```python
from build123d import *

# Parameters (mm, degrees)
SKETCH_W        = 65
SKETCH_H        = 32
SKETCH_R        = 1.75
SKETCH_W_2      = 28
SKETCH_H_2      = 20
SKETCH_W_3      = 15.3
SKETCH_H_3      = 21
PAD_DEPTH       = 14
SKETCH001_W     = 63
SKETCH001_H     = 30
POCKET_DEPTH    = 11
SKETCH002_W     = 6.174751
SKETCH002_H     = 9.5
POCKET001_DEPTH = 7
SKETCH004_W     = 2
SKETCH004_H     = 20
PAD001_DEPTH    = 2
SKETCH005_W     = 15
SKETCH005_H     = 4
POCKET002_DEPTH = 5
SKETCH003_W     = 53
SKETCH003_H     = 5.2
POCKET003_DEPTH = 32.0010000001


with BuildPart() as part:
    # Sketch → Pad (new body)
    with BuildSketch(Plane.XY):
        with Locations((32.5, 16)):
            Rectangle(SKETCH_W, SKETCH_H)
        with Locations((3.5, 28.5)):
            Circle(SKETCH_R, mode=Mode.SUBTRACT)
        with Locations((61.4999634499, 28.5)):
            Circle(SKETCH_R, mode=Mode.SUBTRACT)
        with Locations((3.5, 3.5)):
            Circle(SKETCH_R, mode=Mode.SUBTRACT)
        with Locations((61.4999634499, 3.5)):
            Circle(SKETCH_R, mode=Mode.SUBTRACT)
        with Locations((41.4999634499, 16.7655958753)):
            Rectangle(SKETCH_W_2, SKETCH_H_2, mode=Mode.SUBTRACT)
        with Locations((14.8499634499, 17.4539391628)):
            Rectangle(SKETCH_W_3, SKETCH_H_3, mode=Mode.SUBTRACT)
    extrude(amount=PAD_DEPTH)

    # Sketch001 → Pocket (cut)
    with BuildSketch(Plane(origin=(0, 0, 0), x_dir=(1, 0, 0), z_dir=(0, 0, -1))):
        with Locations((32.5, -16)):
            Rectangle(SKETCH001_W, SKETCH001_H)
    extrude(amount=-POCKET_DEPTH, mode=Mode.SUBTRACT)

    # Sketch002 → Pocket001 (cut)
    with BuildSketch(Plane.XY.offset(14)):
        with Locations((61.9126245, 16)):
            Rectangle(SKETCH002_W, SKETCH002_H)
    extrude(amount=-POCKET001_DEPTH, mode=Mode.SUBTRACT)

    # Sketch004 → Pad001 (new body)
    with BuildSketch(Plane(origin=(0, 0, 11), x_dir=(1, 0, 0), z_dir=(0, 0, -1))):
        with Locations((26.4999634499, -16.7655958753)):
            Rectangle(SKETCH004_W, SKETCH004_H)
        with Locations((56.4999634499, -16.7655958753)):
            Rectangle(SKETCH004_W, SKETCH004_H)
    extrude(amount=PAD001_DEPTH)

    # Sketch005 → Pocket002 (cut)
    with BuildSketch(Plane(origin=(0, 0, 0), x_dir=(0, -1, 0), z_dir=(-1, 0, 0))):
        with Locations((-15.5, 5)):
            Rectangle(SKETCH005_W, SKETCH005_H)
    extrude(amount=-POCKET002_DEPTH, mode=Mode.SUBTRACT)

    # Sketch003 → Pocket003 (cut, through all)
    with BuildSketch(Plane(origin=(0, 32, 0), x_dir=(-1, 0, 0), z_dir=(0, 1, 0))):
        with Locations((-32.5, 6.4)):
            Rectangle(SKETCH003_W, SKETCH003_H)
    extrude(amount=-POCKET003_DEPTH, mode=Mode.SUBTRACT)


solid = part.part
```
Read the model definition and answer for the solid it produces. Units are mm, in the model's axes. A direction names the side the tool comes from. Give positions to 0.01 mm unless a question says otherwise; leave off trailing zeros. Order: outer loops, then holes, each group sorted by start corner. A loop starts at its lowest first (then second) coordinate and runs counter-clockwise, first axis right, second up. Notation, with made-up numbers: (21.5, 72.25) -> (75.5, 72.25) arc R18 ccw to (75.5, 84.25) -> close; hole circle Ø3 at (76, 21). An arc over 180 degrees is marked (long way). Write item = value, one per line.
1. For faces 1 (the face through (26, 6.766, 10)), 2 (the face through (22.5, 17, 12)), 3 (the face through (56, 17, 9)), determine the directions among +Z, -Z, +X, -X, +Y, -Y from which every point of the face is accessible in a straight line to the end or side of a thin tool.
Numbers:
face_1 = -Z
face_2 = +Z, -Z
face_3 = -Z, +Y, -Y
2. Given pin 1 (4.5 mm diameter, centred on x = 3.5, y = 28.5, fed in from -Z); pin 2 (8 mm diameter, centred on x = 31.5, z = 6.5, fed in from +Y); pin 3 (2 mm diameter, centred on x = 56.5, y = 12, fed in from -Z), each flat-ended and moving along its own axis, determine where each tip first touches the part or whether it passes through.
Numbers:
pin_1 = 11
pin_2 = 32
pin_3 = 9
3. A cutting plane is placed at A-A, the plane x = 14. Write down the section's boundary in (y, z), and give its area (3 significant figures).
Numbers:
outline = (0, 0) -> (1, 0) -> (1, 3.8) -> (0, 3.8) -> close; (0, 9) -> (1, 9) -> (1, 11) -> (6.95, 11) -> (6.95, 14) -> (0, 14) -> close; (27.95, 11) -> (31, 11) -> (31, 9) -> (32, 9) -> (32, 14) -> (27.95, 14) -> close; (31, 0) -> (32, 0) -> (32, 3.8) -> (31, 3.8) -> close
area = 44.6 mm²
4. The mould has two halves that part along Y. Classify faces 4 (the face through (32, 32, 10)), 5 (the face through (0, 16, 8)), 6 (the face through (7.2, 17, 12)): +Y half, -Y half, draft (parallel to the pull), parting line (faces both ways), or undercut.
Numbers:
face_4 = +Y half
face_5 = draft
face_6 = undercut
5. Straight lines are drawn through the part: line 1 along X through (y, z) = (3.5, 13.35); line 2 along X through (y, z) = (9, 11.5); line 3 along Y through (x, z) = (3.5, 12.75). For each, find the intervals that lie inside material, in ascending order.
Numbers:
line_1 = 0 to 1.75, 5.25 to 59.75, 63.25 to 65
line_2 = 0 to 7.2, 22.5 to 27.5, 55.5 to 65
line_3 = 0 to 1.75, 5.25 to 26.75, 30.25 to 32
6. A cutting plane is placed at D-D, the plane z = 6. Write down the section's boundary in (x, y), and give its area (3 significant figures).
Numbers:
outline = (0, 0) -> (6, 0) -> (6, 1) -> (1, 1) -> (1, 8) -> (0, 8) -> close; (0, 23) -> (1, 23) -> (1, 31) -> (6, 31) -> (6, 32) -> (0, 32) -> close; (59, 0) -> (65, 0) -> (65, 32) -> (59, 32) -> (59, 31) -> (64, 31) -> (64, 1) -> (59, 1) -> close
area = 69.0 mm²
7. A cutting plane is placed at B-B, the plane y = 3.5. Write down the section's boundary in (x, z).
Numbers:
outline = (0, 0) -> (1, 0) -> (1, 11) -> (1.75, 11) -> (1.75, 14) -> (0, 14) -> close; (5.25, 11) -> (59.75, 11) -> (59.75, 14) -> (5.25, 14) -> close; (63.25, 11) -> (64, 11) -> (64, 0) -> (65, 0) -> (65, 14) -> (63.25, 14) -> close
8. A cutting plane is placed at C-C, the plane y = 9.5. Write down the section's boundary in (x, z).
Numbers:
outline = (0, 0) -> (1, 0) -> (1, 3) -> (0, 3) -> close; (0, 7) -> (1, 7) -> (1, 11) -> (7.2, 11) -> (7.2, 14) -> (0, 14) -> close; (22.5, 11) -> (25.5, 11) -> (25.5, 9) -> (27.5, 9) -> (27.5, 14) -> (22.5, 14) -> close; (55.5, 9) -> (57.5, 9) -> (57.5, 11) -> (64, 11) -> (64, 0) -> (65, 0) -> (65, 14) -> (55.5, 14) -> close
